Study the drawing (mm; zero at the part's minimum x, y, z) and answer. A direction names the side the tool comes from. Round coordinates to 2 decimals unless told otherwise and drop trailing zeros. Loops run counter-clockwise (first coordinate to the right, second up) from the corner with the lowest first, then second, coordinate; pieces in that order, holes last. Notation, with made-up numbers: (52, -13.75) - (73, -13.75) arc R10 cw to (73, 3.25) - close; hole circle Ø6 at (44.5, -27). An arc over 180 degrees is marked (long way). One line per item, written item: value.
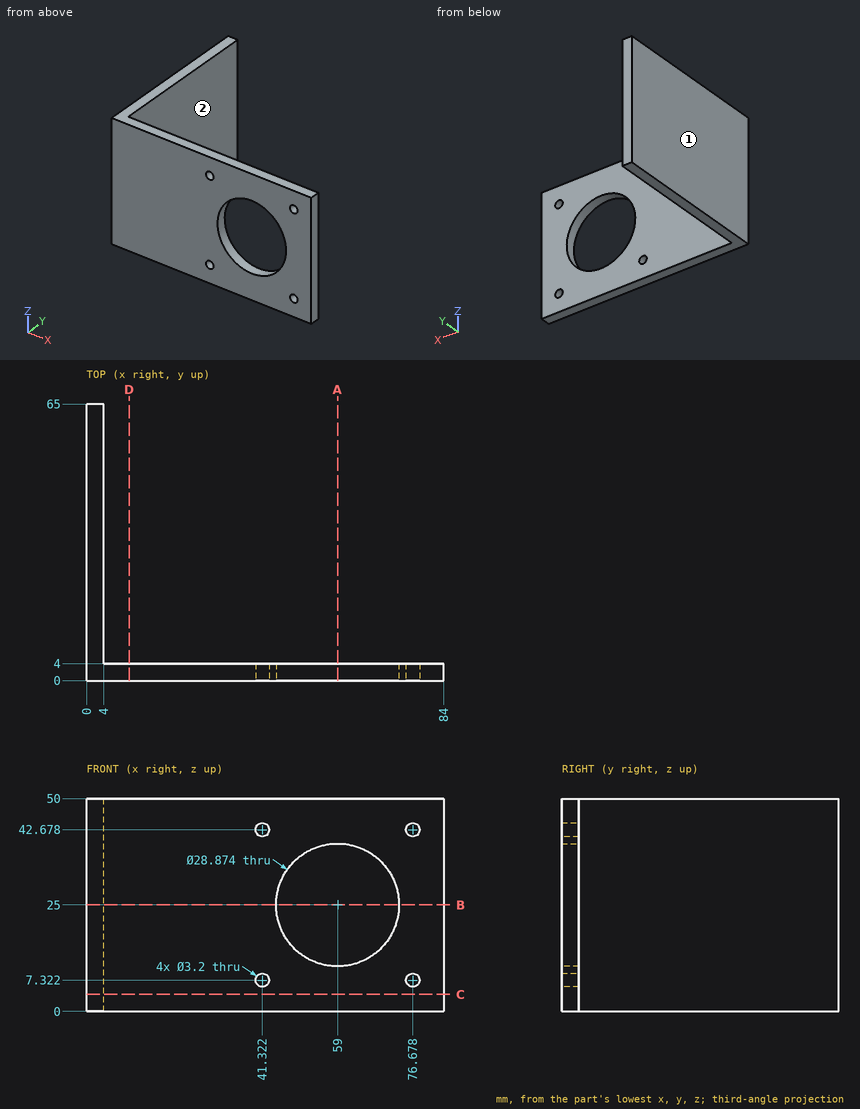
1) Each of these flat-tipped pins is pushed along its axis until it touches: pin 1 Ø6 at (y, z) = (31, 18) entering from +X; pin 2 Ø23 at (x, z) = (59, 25) entering from -Y; pin 3 Ø5 at (x, z) = (21, 42) entering from +Y. Where does it stop, or does it pass through?
Final values:
pin 1: x = 4
pin 2: through
pin 3: y = 4
2) Consider L1, parallel to X at y = 48.5, z = 6; L2, parallel to X at y = 2, z = 25. Determine where each line is inside the solid, lowest interval first.
Final values:
L1: 0 to 4
L2: 0 to 44.56, 73.44 to 84
3) A cutting plane is placed at A-A on x = 59. Give the vertices of the cut face in (y, z), and give its area (3 significant figures).
Final values:
outline: (0, 0) - (4, 0) - (4, 10.56) - (0, 10.56) - close; (0, 39.44) - (4, 39.44) - (4, 50) - (0, 50) - close
area: 84.5 mm2
4) For the marked faces 1 and 2, determine the directions among +Z, -Z, +X, -X, +Y, -Y from which every point of the face is accessible in a straight line to the end or side of a thin tool.
Final values:
face 1: +Z, -Z, -X, +Y, -Y
face 2: +Z, -Z, +X, +Y
5) A cutting plane is placed at C-C on z = 4. Give the vertices of the cut face in (x, y).
Final values:
outline: (0, 0) - (84, 0) - (84, 4) - (4, 4) - (4, 65) - (0, 65) - close
6) A cutting plane is placed at B-B on z = 25. Give the vertices of the cut face in (x, y).
Final values:
outline: (0, 0) - (44.56, 0) - (44.56, 4) - (4, 4) - (4, 65) - (0, 65) - close; (73.44, 0) - (84, 0) - (84, 4) - (73.44, 4) - close
7) A cutting plane is placed at D-D on x = 10. Give the vertices of the cut face in (y, z).
Final values:
outline: (0, 0) - (4, 0) - (4, 50) - (0, 50) - close
